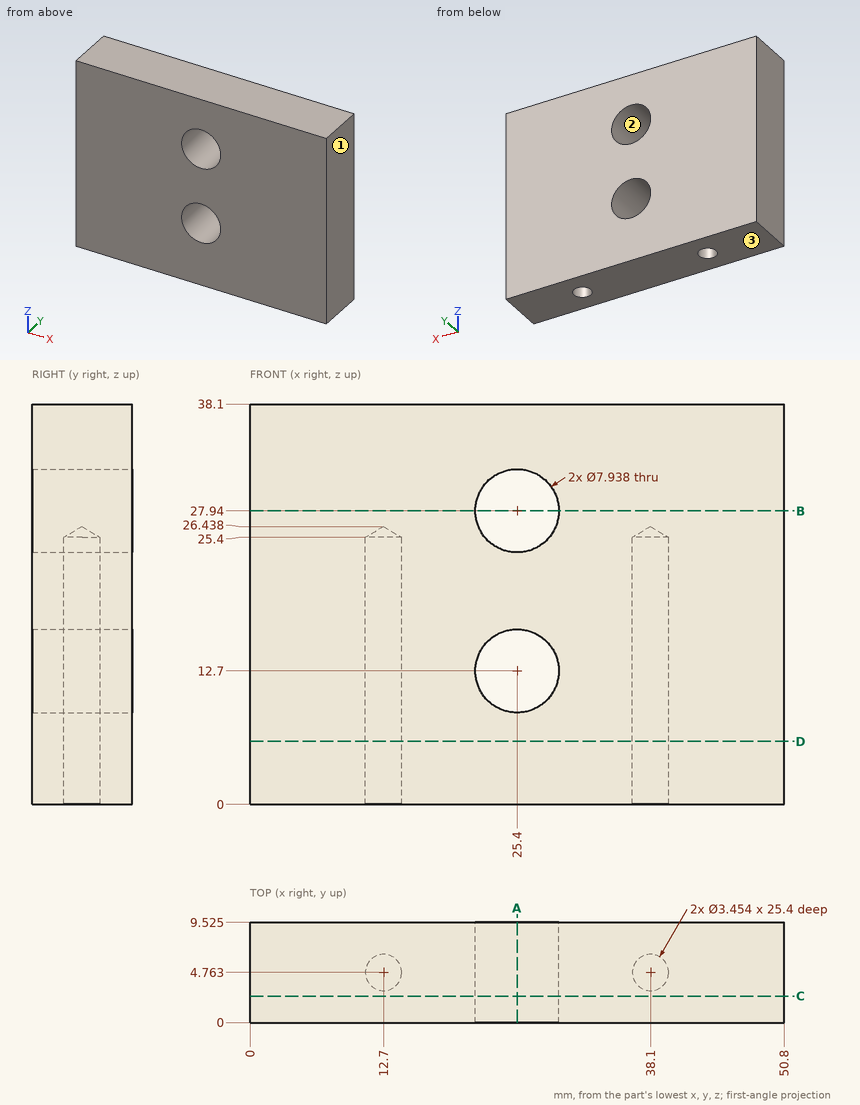
Here's the drawing with two shaded views (mm, measured from the low corner). I have some questions. Coordinates: 2 decimals unless noted, no trailing zeros. Loops run counter-clockwise (first coordinate to the right, second up) from the corner with the lowest first, then second, coordinate; pieces in that order, holes last. Notation, with made-up numbers: M 28,58.5 L 41,58.5 A13 cw 41,76.5 Z; hole C -24,9.25 d1. An arc over 180 degrees is marked long. Answer as CSV lines item,"result". Start each with the question number.
1. Suppose I cut it at D-D, the plane z = 6. List the corners of the cut face in (x, y) for me (1 decimal).
2. Thinking about a two-plate mould opening in Z: for the marked faces 1, 2 and 3, which applies, +Z half, -Z half, draft (parallel to the pull), parting line (faces both ways), or undercut?
3. Suppose I cut it at A-A, the plane x = 25.4. List the corners of the cut face in (y, z) for me (1 decimal), plus the area to 3 significant figures.
4. If I drill on probe 1 along Z at (x, y) = (25.4, 7.5); probe 2 along Y at (x, z) = (38, 9) (1 decimal); probe 3 along Z at (x, y) = (24.5, 7.25) (1 decimal), over which ranges is the centre line in solid material (lowest first)? Write a range as [from, to].
5. For pin 1 Ø5 at (y, z) = (4.5, 13) entering from -X, with a flat end and sliding along its axis, tell me the tip position at first contact or that it passes through.
6. Suppose I cut it at C-C, the plane y = 2.5. List the corners of the cut face in (x, z) for me, plus the area to 3 significant figures.
7. Suppose I cut it at B-B, the plane z = 27.94. List the corners of the cut face in (x, y) for me (1 decimal).
Output:
1,outline,"M 0,0 L 50.8,0 L 50.8,9.5 L 0,9.5 Z; hole C 12.7,4.8 d3.5; hole C 38.1,4.8 d3.5"
2,face 1,"draft"
2,face 2,"undercut"
2,face 3,"-Z half"
3,outline,"M 0,0 L 9.5,0 L 9.5,8.7 L 0,8.7 Z; M 0,16.7 L 9.5,16.7 L 9.5,24 L 0,24 Z; M 0,31.9 L 9.5,31.9 L 9.5,38.1 L 0,38.1 Z"
3,area,"212 mm^2"
4,probe 1,"z = [0, 8.73], [16.67, 23.97], [31.91, 38.1]"
4,probe 2,"y = [0, 3], [6.5, 9.5]"
4,probe 3,"z = [0, 8.8], [16.6, 24.1], [31.8, 38.1]"
5,pin 1,"stops at x = 0"
6,outline,"M 0,0 L 50.8,0 L 50.8,38.1 L 0,38.1 Z; hole C 25.4,12.7 d7.94; hole C 25.4,27.94 d7.94"
6,area,"1,840 mm^2"
7,outline,"M 0,0 L 21.4,0 L 21.4,9.5 L 0,9.5 Z; M 29.4,0 L 50.8,0 L 50.8,9.5 L 29.4,9.5 Z"
